Input: part model. Units: mm. Frame: model coordinates. Round coordinates to 2 decimals unless told otherwise and drop trailing zeros. Loops run counter-clockwise (first coordinate to the right, second up) from the corner with the lowest first, then second, coordinate; pieces in that order, holes last.
1) Section A-A, the plane x = 0. Return loops of the section in (y, z).
2) Section B-B, the plane z = 168. Return loops of the section in (x, y), and give its area (3 significant figures).
3) First-contact query: pin 1 (10 mm diameter, centred on x = 9, z = 109, fed in from +Y); pin 2 (8 mm diameter, centred on x = 4.5, z = 143, fed in from -Y); pin 3 (2 mm diameter, centred on y = 7.5, z = 75.5, fed in from -X). Flat tips, straight axial feed; report the tip coordinate or a pass-through.
4) Draft query along Y for faces 1 (the face through (-2.75, -12.4, 272.94)), 2 (the face through (11.2, -3.7, 0)), 3 (the face through (5.36, -10.31, 272.94)). Return one class per face: pulls with the +Y half, pulls with the -Y half, needs draft (parallel to the pull), parting line crosses it, or undercut.
5) Ray query, line 1 along Z through (x, y) = (12.2, 0); line 2 along Y through (x, z) = (0, 381); line 3 along X through (y, z) = (9.75, 432). Return the intervals inside material, ascending.
from build123d import *

# Parameters (mm, degrees)
SKETCH1_R           = 12.7
SKETCH1_R_2         = 11.6205
BOSS_EXTRUDE1_DEPTH = 553.63
SKETCH3_W           = 1.2
SKETCH3_H           = 12.7


with BuildPart() as part:
    # Sketch1 → Boss-Extrude1 (new body)
    with BuildSketch(Plane.XY):
        Circle(SKETCH1_R)
        Circle(SKETCH1_R_2, mode=Mode.SUBTRACT)
    extrude(amount=BOSS_EXTRUDE1_DEPTH)

    # Sketch3 → M2 Clearance Hole1 (revolve, cut)
    with BuildSketch(Plane(origin=(0, 0, 9), x_dir=(0, 0, 1), z_dir=(0, 1, 0))):
        with Locations((0.6, 6.35)):
            Rectangle(SKETCH3_W, SKETCH3_H)
    m2_clearance_hole1 = revolve(axis=Axis((-6.35, 0, 9), (1, 0, 0)), mode=Mode.SUBTRACT)

    # Mirror1: M2 Clearance Hole1 across plane
    add(m2_clearance_hole1.mirror(Plane(origin=(0, 0, 0), x_dir=(0, 0, 1), z_dir=(1, 0, 0))), mode=Mode.SUBTRACT)


solid = part.part
Final values:
1. outline: (-12.7, 0) - (-11.62, 0) - (-11.62, 553.63) - (-12.7, 553.63) - close; (11.62, 0) - (12.7, 0) - (12.7, 553.63) - (11.62, 553.63) - close
2. outline: circle Ø25.4 at (0, 0); hole circle Ø23.24 at (0, 0)
2. area: 82.5 mm2
3. pin 1: stops at y = 12.05
3. pin 2: stops at y = -12.69
3. pin 3: stops at x = -10.91
4. face 1: parting line crosses it
4. face 2: needs draft
4. face 3: undercut
5. line 1: z = 0 to 7.8, 10.2 to 553.63
5. line 2: y = -12.7 to -11.62, 11.62 to 12.7
5. line 3: x = -8.14 to -6.32, 6.32 to 8.14
